Source: CAD feature listing. Evaluate the final solid. Frame: model axes, mm. A direction names the side the tool comes from. Give positions to 0.01 mm unless a question says otherwise; leave off trailing zeros. Write each loop counter-clockwise with the first axis right and the second up, starting at its lowest first coordinate (ties: lowest second). Pieces come first, ordered by that corner, then holes. Notation, with made-up numbers: (71, 36) -> (94, 36) arc R20 cw to (94, 57) -> close; hole circle Ø11 at (36, -14.5). An arc over 180 degrees is marked (long way). Use one line per item in the form item = value. Start each with the question number.
(1) Material intervals for line 1 along X through (y, z) = (-4.5, 995.5); line 2 along Y through (x, z) = (63, 427), sorted ascending. Write a range as from..to.
(2) Draft query along X for faces 3 (the face through (-65, -3, 608)), 4 (the face through (-0.3, 20.5, 1200)), 5 (the face through (70, -3, 592)). Return one class per face: pulls with the +X half, pulls with the -X half, needs draft (parallel to the pull), parting line crosses it, or undercut.
(3) Cut plane A-A, the plane y = 5.5. Output: boundary loops of the cut face in (x, z), and give its area (3 significant figures).
(4) Set-up query: faces 1 (the face through (-0.3, 20.5, 0)), 2 (the face through (65, -3, 608)). Return all of +Z, -Z, +X, -X, +Y, -Y with unobstructed straight access to the full face (end or side cutting, diameter ignored); none if empty.
(5) Cut plane C-C, the plane x = -53. Output: boundary loops of the cut face in (y, z), and give its area (3 significant figures).
(6) First-contact query: P1, Ø1, axis at x = 33.5, z = 1038, coming from the -Y side. Flat tip, straight axial feed; report the tip coordinate or a pass-through.
(7) Cut plane B-B, the plane z = 364. Output: boundary loops of the cut face in (x, y).
from build123d import *

# Parameters (mm, degrees)
ESBO_O1_W                = 140
ESBO_O1_H                = 50
RESSALTO_EXTRUS_O1_DEPTH = 1200
FILETE1_R                = 5
CASCA1_START             = -65
CASCA1_OUTLINE_W         = 45
CASCA1_OUTLINE_H         = 1200
CASCA1_DEPTH             = 130


# Read off the part's stored shape, not the designer's step: Casca1
with BuildPart() as part:
    # Esboço1 → Ressalto-extrusão1 (new body)
    with BuildSketch(Plane.XY):
        Rectangle(ESBO_O1_W, ESBO_O1_H)
    extrude(amount=RESSALTO_EXTRUS_O1_DEPTH)

    # Filete1
    filete1_edges = [part.edges().sort_by_distance(p)[0] for p in [
        (-70, 25, 600),
        (70, 25, 600),
    ]]
    fillet(filete1_edges, radius=FILETE1_R)

    # Casca1 outline → Casca1 (cut)
    with BuildSketch(Plane.YZ.offset(CASCA1_START)):
        with Locations((-2.5, 600)):
            Rectangle(CASCA1_OUTLINE_W, CASCA1_OUTLINE_H)
    extrude(amount=CASCA1_DEPTH, mode=Mode.SUBTRACT)


solid = part.part
Geometry says:
q1.line_1 = -70..-65, 65..70
q1.line_2 = 20..25
q2.face_3 = undercut
q2.face_4 = needs draft
q2.face_5 = pulls with the +X half
q3.outline = (-70, 0) -> (-65, 0) -> (-65, 1200) -> (-70, 1200) -> close; (65, 0) -> (70, 0) -> (70, 1200) -> (65, 1200) -> close
q3.area = 12,000 mm^2
q4.face_1 = -Z, +X, -X, +Y, -Y
q4.face_2 = +Z, -Z, -Y
q5.outline = (20, 0) -> (25, 0) -> (25, 1200) -> (20, 1200) -> close
q5.area = 6,000 mm^2
q6.P1 = 20
q7.outline = (-70, -25) -> (-65, -25) -> (-65, 20) -> (65, 20) -> (65, -25) -> (70, -25) -> (70, 20) arc R5 ccw to (65, 25) -> (-65, 25) arc R5 ccw to (-70, 20) -> close
